Verification items for the finished model (mm, model axes). A direction names the side the tool comes from. Give positions to 0.01 mm unless a question says otherwise; leave off trailing zeros. Loops run counter-clockwise (first coordinate to the right, second up) from the corner with the lowest first, then second, coordinate; pieces in that order, holes last. Notation, with made-up numbers: M -26,-8.75 L -16,-8.75 A23 cw -16,17.25 Z; hole C 25,57.5 d6. An arc over 180 degrees is marked long. Put each result on its own line as item: value. Start each with the question number.
from build123d import *

# Parameters (mm, degrees)
F2_DEPTH = 25
F3_R     = 4.5
F4_DEPTH = 3
F5_R     = 4.5
F6_DEPTH = 3


with BuildPart() as f2:
    # F1 (on Top) → F2 (new body)
    with BuildSketch(Plane.XY):
        Polygon((-31, 0), (0, 0), (0, 31), (-3, 31), (-3, 3), (-31, 3), align=None)
    extrude(amount=F2_DEPTH)

    # F3 (on face) → F4 (cut, through all)
    with BuildSketch(Plane.XZ):
        with Locations((-21.5, 12.5)):
            Circle(F3_R)
    extrude(amount=-F4_DEPTH, mode=Mode.SUBTRACT)

    # F5 (on face) → F6 (cut, through all)
    with BuildSketch(Plane.YZ):
        with Locations((21.5, 12.5)):
            Circle(F5_R)
    extrude(amount=-F6_DEPTH, mode=Mode.SUBTRACT)


solid = f2.part
Q1. Set-up check for faces 4 (the face through (-9, 2, 0)), 5 (the face through (-16.8, 3, 12.3)): record each of +Z, -Z, +X, -X, +Y, -Y from which the full face is reachable in a straight line by a thin tool's end or side.
Q2. Go/stop test with flat-tipped pins: pin 1 (2 mm diameter, centred on x = -14.5, z = 12, fed in from -Y); pin 2 (10.5 mm diameter, centred on y = 21.5, z = 12.5, fed in from -X). Record where each tip stops, or that it passes through.
Q3. Cross-section at B-B, the plane x = -21.5. Record the boundary of the cut face in (y, z), then the cut area to 3 significant figures.
Q4. Cross-section at C-C, the plane y = 21.5. Record the boundary of the cut face in (x, z), then the cut area to 3 significant figures.
Q5. Cross-section at D-D, the plane x = -2.5. Record the boundary of the cut face in (y, z), then the cut area to 3 significant figures.
Q6. Scan lines: L1, parallel to Z at x = -2.2, y = 21.5; L2, parallel to X at y = 13, z = 10.25; L3, parallel to Y at x = -15, z = 3.25. Record each from-to range of solid material in increasing order.
Q7. Release check for a two-part mould opening along Y. For faces 1 (the face through (-1, 31, 12)), 2 (the face through (-31, 2, 12)), 3 (the face through (-1.479, 17.004, 12.698)) record: pulls with the +Y half, pulls with the -Y half, needs draft (parallel to the pull), parting line crosses it, or undercut.
Q8. Cross-section at A-A, the plane z = 12.5. Record the boundary of the cut face in (x, y).
Ans:
1. face 4: -Z, +X, -X, +Y, -Y
1. face 5: +Z, -Z, -X, +Y
2. pin 1: stops at y = 0
2. pin 2: stops at x = -3
3. outline: M 0,0 L 3,0 L 3,8 L 0,8 Z; M 0,17 L 3,17 L 3,25 L 0,25 Z
3. area: 48.0 mm^2
4. outline: M -3,0 L 0,0 L 0,8 L -3,8 Z; M -3,17 L 0,17 L 0,25 L -3,25 Z
4. area: 48.0 mm^2
5. outline: M 0,0 L 31,0 L 31,25 L 0,25 Z; hole C 21.5,12.5 d9
5. area: 711 mm^2
6. L1: z = 0 to 8, 17 to 25
6. L2: x = -3 to 0
6. L3: y = 0 to 3
7. face 1: pulls with the +Y half
7. face 2: needs draft
7. face 3: undercut
8. outline: M -31,0 L -26,0 L -26,3 L -31,3 Z; M -17,0 L 0,0 L 0,17 L -3,17 L -3,3 L -17,3 Z; M -3,26 L 0,26 L 0,31 L -3,31 Z
